Design review of the part built by this model. Coordinates are the model's own, in mm. A direction names the side the tool comes from. Give positions to 0.01 mm unless a question says otherwise; leave off trailing zeros. Loops run counter-clockwise (first coordinate to the right, second up) from the corner with the lowest first, then second, coordinate; pieces in that order, holes last. Notation, with made-up numbers: M 82,9.25 L 89,9.25 A17 cw 89,16.25 Z; hole C -12,10.25 d1. An arc over 180 degrees is marked long. Use a Markdown table: item, result. Add a question column.
(1) Add section A-A, the plane y = 27. Give the boundary of the cut face in (x, z), then the cut area to 3 significant figures.
(2) Add section C-C, the plane y = 12.5. Give the boundary of the cut face in (x, z).
(3) Add section B-B, the plane x = 0. Give the boundary of the cut face in (y, z).
(4) For probe 1 along Y at (x, z) = (2.25, -1.5); probe 2 along X at (y, z) = (9.5, -1); probe 3 along Z at (x, y) = (-0.75, 1), list the stretches that pass through material, from the lowest coordinate up.
(5) Insertion check: pin 1 Ø3 at (x, y) = (3, 9) entering from -Z. The pin has a flat end and moves straight along its axis. Give the tip position at first contact, or say it passes through.
(6) For faces 1 (the face through (-0.29, 12.32, -2.23)), 2 (the face through (0, 27, 3.5)), list the 3-axis set-ups (+Z, -Z, +X, -X, +Y, -Y) from which the entire face can be reached by the end or side of a thin tool; tool diameter is ignored.
```python
from build123d import *

# Parameters (mm, degrees)
SKETCH1_R           = 2.25
BOSS_EXTRUDE1_DEPTH = 25
BOSS_EXTRUDE2_DEPTH = 4
SKETCH3_OUTSIDE_W   = 24.264
SKETCH3_OUTSIDE_H   = 23.182
SKETCH3_OUTSIDE_R   = 3.25
CUT_EXTRUDE1_DEPTH  = 4
CUT_EXTRUDE1_TAPER  = 45


with BuildPart() as part:
    # Sketch1 → Boss-Extrude1 (new body)
    with BuildSketch(Plane(origin=(0, 0, 0), x_dir=(1, 0, 0), z_dir=(0, 1, 0))):
        Circle(SKETCH1_R)
    extrude(amount=BOSS_EXTRUDE1_DEPTH)

    # Sketch2 → Boss-Extrude2 (add)
    with BuildSketch(Plane(origin=(0, 25, 0), x_dir=(1, 0, 0), z_dir=(0, 1, 0))):
        Polygon((4.041451884, 0), (2.020725942, 3.5), (-2.020725942, 3.5), (-4.041451884, 0), (-2.020725942, -3.5), (2.020725942, -3.5), align=None)
    extrude(amount=BOSS_EXTRUDE2_DEPTH)

    # Sketch3 outside → Cut-Extrude1 (cut)
    with BuildSketch(Plane(origin=(0, 29, 0), x_dir=(1, 0, 0), z_dir=(0, 1, 0))):
        Rectangle(SKETCH3_OUTSIDE_W, SKETCH3_OUTSIDE_H)
        Circle(SKETCH3_OUTSIDE_R, mode=Mode.SUBTRACT)
    extrude(amount=-CUT_EXTRUDE1_DEPTH, taper=CUT_EXTRUDE1_TAPER, mode=Mode.SUBTRACT)


solid = part.part
```
Established:
| question | item | result |
|---|---|---|
| 1 | outline | M -4.04,0 L -2.02,-3.5 L 2.02,-3.5 L 4.04,0 L 2.02,3.5 L -2.02,3.5 Z |
| 1 | area | 42.4 mm^2 |
| 2 | outline | C 0,0 d4.5 |
| 3 | outline | M 0,-2.25 L 25,-2.25 L 25,-3.5 L 28.75,-3.5 L 29,-3.25 L 29,3.25 L 28.75,3.5 L 25,3.5 L 25,2.25 L 0,2.25 Z |
| 4 | probe 1 | 25 to 29 |
| 4 | probe 2 | -2.02 to 2.02 |
| 4 | probe 3 | -2.12 to 2.12 |
| 5 | pin 1 | z = -1.68 |
| 6 | face 1 | -Y |
| 6 | face 2 | +Z, +X, -X, +Y, -Y |
